```python
from build123d import *

# Parameters (mm, degrees)
SKETCH1_R           = 9.75
SKETCH1_R_2         = 2.25
SKETCH1_R_3         = 1.5
BOSS_EXTRUDE1_DEPTH = 4.5
SKETCH2_R           = 1.5
CUT_EXTRUDE1_DEPTH  = 15.504309704
SKETCH3_R           = 2.75
CUT_EXTRUDE2_DEPTH  = 3


with BuildPart() as part:
    # Sketch1 → Boss-Extrude1 (new body)
    with BuildSketch(Plane.XY):
        Circle(SKETCH1_R)
        Circle(SKETCH1_R_2, mode=Mode.SUBTRACT)
        with Locations((0, 6)):
            Circle(SKETCH1_R_3, mode=Mode.SUBTRACT)
        with Locations((6, 0)):
            Circle(SKETCH1_R_3, mode=Mode.SUBTRACT)
        with Locations((0, -6)):
            Circle(SKETCH1_R_3, mode=Mode.SUBTRACT)
        with Locations((-6, 0)):
            Circle(SKETCH1_R_3, mode=Mode.SUBTRACT)
    extrude(amount=BOSS_EXTRUDE1_DEPTH)

    # Sketch2 → Cut-Extrude1 (cut, through all)
    with BuildSketch(Plane.XY.offset(4.5)):
        with Locations((2.298097039, 2.298097039)):
            Circle(SKETCH2_R)
        with Locations((-2.298097039, -2.298097039)):
            Circle(SKETCH2_R)
    extrude(amount=-CUT_EXTRUDE1_DEPTH, mode=Mode.SUBTRACT)

    # Sketch3 → Cut-Extrude2 (cut)
    with BuildSketch(Plane.XY.offset(4.5)):
        with Locations((6, 0)):
            Circle(SKETCH3_R)
        with Locations((0, -6)):
            Circle(SKETCH3_R)
        with Locations((-6, 0)):
            Circle(SKETCH3_R)
        with Locations((0, 6)):
            Circle(SKETCH3_R)
    extrude(amount=-CUT_EXTRUDE2_DEPTH, mode=Mode.SUBTRACT)


solid = part.part
```
Check sheet for the modelled part. Datum: model origin and axes. Units: mm. A direction names the side the tool comes from. Give positions to 0.01 mm unless a question says otherwise; leave off trailing zeros. Order: outer loops, then holes, each group sorted by start corner. A loop starts at its lowest first (then second) coordinate and runs counter-clockwise, first axis right, second up. Notation, with made-up numbers: (-5, 61.25) -> (53, 61.25) arc R31 cw to (53, 95.25) -> close; hole circle Ø8 at (29, -11). An arc over 180 degrees is marked (long way). Use CSV: the item, a comma, the result in double quotes. Start each with the question number.
1) Sectioned sample at A-A, the plane x = 4.75. Record the boundary of the cut face in (y, z).
2) Sectioned sample at C-C, the plane y = -7. Record the boundary of the cut face in (x, z).
3) Material ranges on line 1 (Y direction, x = 0, z = 3.55); line 2 (Y direction, x = 3.5, z = 3.45); line 3 (X direction, y = 1, z = 0.55), recorded low to high. Write a range as from..to.
4) Sectioned sample at B-B, the plane y = 0. Record the boundary of the cut face in (x, z), plus the area to 3 significant figures.
5) Sectioned sample at D-D, the plane x = -0.25. Record the boundary of the cut face in (y, z), plus the area to 3 significant figures.
6) Mould release check, pull along X, two halves, no side actions. Record for faces 1 (the face through (-3.395, -3.321, 2.282)), 2 (the face through (-0.325, -7.464, 0.74)), 3 (the face through (2, -2, 0)), 4 (the face through (-1.269, 9.667, 2.218)): released by +X, released by -X, zero draft, split by the parting line, or undercut.
7) Go/stop test with flat-tipped pins: P1, Ø3, axis at x = -0.5, y = -6.5, coming from the +Z side; P2, Ø1.8, axis at x = 2.3, y = 2.3, coming from the +Z side; P3, Ø1, axis at x = -6.5, z = 1.5, coming from the -Y side; P4, Ø1.5, axis at x = 2, z = 3, coming from the -Y side. Record where each tip stops, or that it passes through.
8) Set-up check for faces 5 (the face through (1.2, 4.8, 1.5)), 6 (the face through (4.8, -0.9, 0.7)): record each of +Z, -Z, +X, -X, +Y, -Y from which the full face is reachable in a straight line by a thin tool's end or side.
Recorded:
1,outline,"(-8.51, 0) -> (-0.83, 0) -> (-0.83, 1.5) -> (-2.45, 1.5) -> (-2.45, 4.5) -> (-8.51, 4.5) -> close; (0.83, 0) -> (8.51, 0) -> (8.51, 4.5) -> (2.45, 4.5) -> (2.45, 1.5) -> (0.83, 1.5) -> close"
2,outline,"(-6.79, 0) -> (-1.12, 0) -> (-1.12, 1.5) -> (-2.56, 1.5) -> (-2.56, 4.5) -> (-6.79, 4.5) -> close; (1.12, 0) -> (6.79, 0) -> (6.79, 4.5) -> (2.56, 4.5) -> (2.56, 1.5) -> (1.12, 1.5) -> close"
3,line 1,"-9.75..-8.75, -3.25..-2.25, 2.25..3.25, 8.75..9.75"
3,line 2,"-9.1..-1.15, 1.15..1.4, 3.2..9.1"
3,line 3,"-9.7..-7.12, -4.88..-2.02, 3.05..4.88, 7.12..9.7"
4,outline,"(-9.75, 0) -> (-7.5, 0) -> (-7.5, 1.5) -> (-8.75, 1.5) -> (-8.75, 4.5) -> (-9.75, 4.5) -> close; (-4.5, 0) -> (-2.25, 0) -> (-2.25, 4.5) -> (-3.25, 4.5) -> (-3.25, 1.5) -> (-4.5, 1.5) -> close; (2.25, 0) -> (4.5, 0) -> (4.5, 1.5) -> (3.25, 1.5) -> (3.25, 4.5) -> (2.25, 4.5) -> close; (7.5, 0) -> (9.75, 0) -> (9.75, 4.5) -> (8.75, 4.5) -> (8.75, 1.5) -> (7.5, 1.5) -> close"
4,area,"25.5 mm2"
5,outline,"(-9.75, 0) -> (-7.48, 0) -> (-7.48, 1.5) -> (-8.74, 1.5) -> (-8.74, 4.5) -> (-9.75, 4.5) -> close; (-4.52, 0) -> (-2.24, 0) -> (-2.24, 4.5) -> (-3.26, 4.5) -> (-3.26, 1.5) -> (-4.52, 1.5) -> close; (2.24, 0) -> (4.52, 0) -> (4.52, 1.5) -> (3.26, 1.5) -> (3.26, 4.5) -> (2.24, 4.5) -> close; (7.48, 0) -> (9.75, 0) -> (9.75, 4.5) -> (8.74, 4.5) -> (8.74, 1.5) -> (7.48, 1.5) -> close"
5,area,"25.9 mm2"
6,face 1,"undercut"
6,face 2,"undercut"
6,face 3,"zero draft"
6,face 4,"split by the parting line"
7,P1,"z = 1.5"
7,P2,"through"
7,P3,"y = -7.69"
7,P4,"y = -9.67"
8,face 5,"+Z"
8,face 6,"+Z, -Z"
